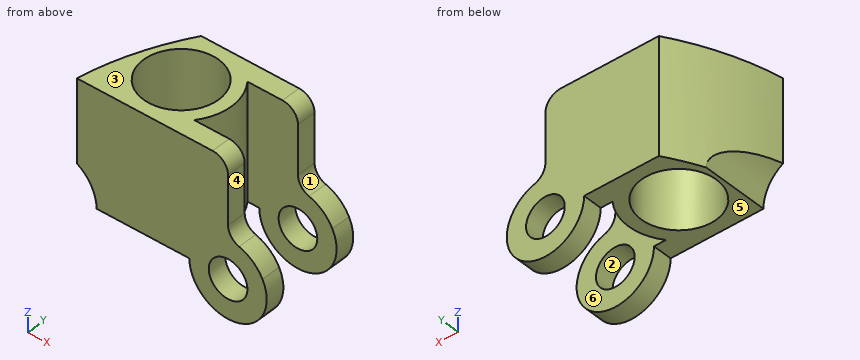
from build123d import *

# Parameters (mm, degrees)
SKETCH2_R           = 6.1595
BOSS_EXTRUDE1_DEPTH = 25.4
SKETCH3_R           = 3.175
CUT_EXTRUDE1_DEPTH  = 25.4
CUT_EXTRUDE2_DEPTH  = 17.51
SKETCH7_R           = 6.35
SKETCH7_R_2         = 3.175
BOSS_EXTRUDE2_DEPTH = 3.175
SKETCH8_R           = 6.35
SKETCH8_R_2         = 3.175
BOSS_EXTRUDE3_DEPTH = 3.175
FILLET1_R           = 2.54
FILLET2_R           = 2.54


with BuildPart() as part:
    # Sketch2 → Boss-Extrude1 (new body)
    with BuildSketch(Plane.XY):
        with BuildLine():
            Line((-37.667011981, 23.60082008), (-13.401813639, 23.60082008))
            Line((-13.401813639, 23.60082008), (-13.401813639, 20.42582008))
            Line((-13.401813639, 20.42582008), (-27.350622089, 20.42582008))
            ThreePointArc((-27.350622089, 20.42582008), (-25.602435825, 15.34582008), (-27.350622089, 10.26582008))
            Line((-27.350622089, 10.26582008), (-13.401813639, 10.26582008))
            Line((-13.401813639, 10.26582008), (-13.401813639, 7.09082008))
            Line((-13.401813639, 7.09082008), (-43.880779056, 7.09082008))
            ThreePointArc((-43.880779056, 7.09082008), (-41.601148791, 15.657168302), (-37.667011981, 23.60082008))
        make_face()
        with Locations((-33.857435825, 15.34582008)):
            Circle(SKETCH2_R, mode=Mode.SUBTRACT)
    extrude(amount=BOSS_EXTRUDE1_DEPTH)

    # Sketch3 → Cut-Extrude1 (cut)
    with BuildSketch(Plane(origin=(0, 23.60082008, 0), x_dir=(1, 0, 0), z_dir=(0, 1, 0))):
        with Locations((-19.05, -6.35)):
            Circle(SKETCH3_R)
    extrude(amount=-CUT_EXTRUDE1_DEPTH, mode=Mode.SUBTRACT)

    # Sketch6 → Cut-Extrude2 (cut, through all)
    with BuildSketch(Plane(origin=(0, 23.60082008, 0), x_dir=(1, 0, 0), z_dir=(0, 1, 0))):
        with BuildLine():
            Line((-40.64, 0), (-46.99, 0))
            ThreePointArc((-46.99, 0), (-51.480128061, -10.840128061), (-40.64, -6.35))
            Line((-40.64, -6.35), (-25.4, -6.35))
            ThreePointArc((-25.4, -6.35), (-14.559871939, -1.859871939), (-19.05, -12.7))
            Line((-19.05, -12.7), (-19.05, -25.4))
            Line((-19.05, -25.4), (-13.401813639, -25.4))
            Line((-13.401813639, -25.4), (-10.329666698, -21.085123092))
            Line((-10.329666698, -21.085123092), (-9.028029261, 2.468316234))
            Line((-9.028029261, 2.468316234), (-25.4, 3.088143584))
            Line((-25.4, 3.088143584), (-40.64, 0))
        make_face()
    extrude(amount=-CUT_EXTRUDE2_DEPTH, mode=Mode.SUBTRACT)

    # Sketch7 → Boss-Extrude2 (add)
    with BuildSketch(Plane(origin=(0, 23.60082008, 0), x_dir=(1, 0, 0), z_dir=(0, 1, 0))):
        with Locations((-19.05, -6.35)):
            Circle(SKETCH7_R)
        with Locations((-19.05, -6.35)):
            Circle(SKETCH7_R_2, mode=Mode.SUBTRACT)
    extrude(amount=-BOSS_EXTRUDE2_DEPTH)

    # Sketch8 → Boss-Extrude3 (add)
    with BuildSketch(Plane.XZ.offset(-7.09082008)):
        with Locations((-19.05, 6.35)):
            Circle(SKETCH8_R)
        with Locations((-19.05, 6.35)):
            Circle(SKETCH8_R_2, mode=Mode.SUBTRACT)
    extrude(amount=-BOSS_EXTRUDE3_DEPTH)

    # Fillet1
    fillet1_edges = [part.edges().sort_by_distance(p)[0] for p in [
        (-19.05, 22.01332008, 12.7),
        (-19.05, 8.67832008, 12.7),
    ]]
    fillet(fillet1_edges, radius=FILLET1_R)

    # Fillet2
    fillet2_edges = [part.edges().sort_by_distance(p)[0] for p in [
        (-19.05, 22.01332008, 25.4),
        (-19.05, 8.67832008, 25.4),
    ]]
    fillet(fillet2_edges, radius=FILLET2_R)


solid = part.part
Check sheet for the modelled part. Datum: model origin and axes. Units: mm. Face numbers are marked on the shaded views. A direction names the side the tool comes from. Coordinates: 2 decimals unless noted, no trailing zeros. Loops run counter-clockwise (first coordinate to the right, second up) from the corner with the lowest first, then second, coordinate; pieces in that order, holes last. Notation, with made-up numbers: (35, 83) -> (46, 83) arc R34 cw to (46, 119) -> close; hole circle Ø5 at (-34, -28). An arc over 180 degrees is marked (long way). Write item = value, one per line. Start each with the question number.
1. Section check C-C on z = 5.25. Record the cut outline in (x, y), then the cut area to 3 significant figures.
2. Material ranges on line 1 (Y direction, x = -24.5, z = 17.5); line 2 (Y direction, x = -37.5, z = 22.5); line 3 (X direction, y = 8.5, z = 5.5), recorded low to high.
3. Section check A-A on x = -32.5. Record the cut outline in (y, z), then the cut area to 3 significant figures.
4. Depth check by flat-ended pin: P1, Ø6, axis at y = 14.5, z = 6, coming from the -X side; P2, Ø7.5, axis at x = -34, y = 17, coming from the -Z side; P3, Ø4, axis at x = -20, y = 20, coming from the +Z side; P4, Ø6, axis at y = 16.5, z = 4, coming from the -X side. Enter the tip coordinate at first touch or a pass-through.
5. Draft check along X on the marked faces 1, 2 and 3. Enter one of: released by +X, released by -X, zero draft, split by the parting line, or undercut.
6. Section check B-B on y = 19.25. Record the cut outline in (x, z), then the cut area to 3 significant figures.
7. Tool access check on the marked faces 4, 5 and 6. Record the directions out of +Z, -Z, +X, -X, +Y, -Y that give a thin tool (end or side, any length) a straight path to the whole face; none if there is none.
Responses:
q1.outline = (-25.3, 7.09) -> (-22.03, 7.09) -> (-22.03, 10.27) -> (-25.3, 10.27) -> close; (-25.3, 20.43) -> (-22.03, 20.43) -> (-22.03, 23.6) -> (-25.3, 23.6) -> close; (-16.07, 7.09) -> (-12.8, 7.09) -> (-12.8, 10.27) -> (-16.07, 10.27) -> close; (-16.07, 20.43) -> (-12.8, 20.43) -> (-12.8, 23.6) -> (-16.07, 23.6) -> close
q1.area = 41.6 mm2
q2.line_1 = 7.09 to 10.27, 20.43 to 23.6
q2.line_2 = 7.09 to 10.38, 20.31 to 23.6
q2.line_3 = -25.34 to -22.11, -15.99 to -12.76
q3.outline = (7.09, 6.35) -> (9.34, 6.35) -> (9.34, 25.4) -> (7.09, 25.4) -> close; (21.35, 6.35) -> (23.6, 6.35) -> (23.6, 25.4) -> (21.35, 25.4) -> close
q3.area = 85.6 mm2
q4.P1 = -41.22
q4.P2 = through
q4.P3 = 25.4
q4.P4 = -40.67
q5.face_1 = released by +X
q5.face_2 = undercut
q5.face_3 = zero draft
q6.outline = (-40.07, 6.35) -> (-38.62, 6.35) -> (-38.62, 25.4) -> (-40.07, 25.4) -> close; (-29.09, 6.35) -> (-26.58, 6.35) -> (-26.58, 25.4) -> (-29.09, 25.4) -> close
q6.area = 75.3 mm2
q7.face_4 = +Z, +X, +Y, -Y
q7.face_5 = -Z, -X, +Y, -Y
q7.face_6 = +Z, -Z, +X
